```python
from build123d import *

# Parameters (mm, degrees)
SKETCH1_W                                = 60
SKETCH1_H                                = 50
BOSS_EXTRUDE1_DEPTH                      = 10
CUT_EXTRUDE1_DEPTH                       = 10
BOSS_EXTRUDE2_REACH                      = 80.74
CBORE_FOR_M3_PAN_HEAD_SCREW1_D           = 3.4
CBORE_FOR_M3_PAN_HEAD_SCREW1_CBORE_D     = 6.5
CBORE_FOR_M3_PAN_HEAD_SCREW1_CBORE_DEPTH = 3.3
M3X0_5_TAPPED_HOLE1_D                    = 2.6
M3X0_5_TAPPED_HOLE1_DEPTH                = 9
M3X0_5_TAPPED_HOLE1_TIP                  = 0.781118805
M3X0_5_TAPPED_HOLE2_D                    = 2.6
M3X0_5_TAPPED_HOLE2_DEPTH                = 9
M3X0_5_TAPPED_HOLE2_TIP                  = 0.781118805


with BuildPart() as part:
    # Sketch1 → Boss-Extrude1 (new body)
    with BuildSketch(Plane(origin=(0, 0, 0), x_dir=(1, 0, 0), z_dir=(0, 1, 0))):
        with Locations((30, 25)):
            Rectangle(SKETCH1_W, SKETCH1_H)
    extrude(amount=BOSS_EXTRUDE1_DEPTH)

    # Sketch2 → Cut-Extrude1 (cut)
    with BuildSketch(Plane(origin=(0, 10, 0), x_dir=(1, 0, 0), z_dir=(0, 1, 0))):
        with BuildLine():
            Line((38, 48), (38, 50))
            Line((38, 50), (44, 50))
            Line((44, 50), (44, 48))
            ThreePointArc((44, 48), (41, 45), (38, 48))
        make_face()
        with BuildLine():
            Line((10, 48), (10, 50))
            Line((10, 50), (16, 50))
            Line((16, 50), (16, 48))
            ThreePointArc((16, 48), (13, 45), (10, 48))
        make_face()
    extrude(amount=-CUT_EXTRUDE1_DEPTH, mode=Mode.SUBTRACT)

    # Sketch3 → Boss-Extrude2 (add, up to next)
    with BuildSketch(Plane(origin=(0, 0, 0), x_dir=(0, 0, -1), z_dir=(1, 0, 0)), mode=Mode.PRIVATE) as boss_extrude2_sk1:
        Polygon((45, 0), (50, 0), (50, 5), (45, 10), align=None)
    boss_extrude2_tool1 = extrude(boss_extrude2_sk1.sketch, amount=BOSS_EXTRUDE2_REACH, mode=Mode.PRIVATE) - part.part
    add(boss_extrude2_tool1.solids().sort_by_distance((0, 3.888889, -47.222222))[0])
    add(boss_extrude2_tool1.solids().sort_by_distance((0, 3.888889, -47.222222))[1])

    # CBORE for M3 Pan Head Screw1 (through all)
    with Locations(Plane(origin=(5, 10, -42), x_dir=(0, 0, 1), z_dir=(0, 1, 0))):
        with Locations((0, 0), (0, 44)):
            CounterBoreHole(CBORE_FOR_M3_PAN_HEAD_SCREW1_D / 2, CBORE_FOR_M3_PAN_HEAD_SCREW1_CBORE_D / 2, CBORE_FOR_M3_PAN_HEAD_SCREW1_CBORE_DEPTH)

    # M3x0.5 Tapped Hole1
    with Locations(Plane(origin=(60, 0, 0), x_dir=(0, 0, -1), z_dir=(1, 0, 0))):
        with Locations((34, 5), (9, 5)):
            Hole(M3X0_5_TAPPED_HOLE1_D / 2, depth=M3X0_5_TAPPED_HOLE1_DEPTH)
            with Locations((0, 0, -(M3X0_5_TAPPED_HOLE1_DEPTH + M3X0_5_TAPPED_HOLE1_TIP / 2))):  # 118° drill point
                Cone(0, M3X0_5_TAPPED_HOLE1_D / 2, M3X0_5_TAPPED_HOLE1_TIP, mode=Mode.SUBTRACT)

    # M3x0.5 Tapped Hole2
    with Locations(Plane.ZY):
        with Locations((-34, 5), (-9, 5)):
            Hole(M3X0_5_TAPPED_HOLE2_D / 2, depth=M3X0_5_TAPPED_HOLE2_DEPTH)
            with Locations((0, 0, -(M3X0_5_TAPPED_HOLE2_DEPTH + M3X0_5_TAPPED_HOLE2_TIP / 2))):  # 118° drill point
                Cone(0, M3X0_5_TAPPED_HOLE2_D / 2, M3X0_5_TAPPED_HOLE2_TIP, mode=Mode.SUBTRACT)


solid = part.part
```
Work out the finished part from the listing and answer in its coordinate system (mm). A direction names the side the tool comes from. Give positions to 0.01 mm unless a question says otherwise; leave off trailing zeros. Loops run counter-clockwise (first coordinate to the right, second up) from the corner with the lowest first, then second, coordinate; pieces in that order, holes last. Notation, with made-up numbers: M 63,88 L 95,88 A22 ccw 95,123 Z; hole C 64,-32 d6. An arc over 180 degrees is marked long. One line per item, written item: value. Start each with the question number.
1. Find the intervals of material crossed by probe 1 along X at (y, z) = (8.05, -42); probe 2 along Z at (x, y) = (57.25, 5); probe 3 along X at (y, z) = (2, -42), in increasing order.
2. Find section B-B (x = 53.5). Give the vertices of the cut face in (y, z).
3. Which of the six approach directions +Z, -Z, +X, -X, +Y, -Y give full straight-line access (tool end or side, diameter ignored) to faces 1 (the face through (30, 0, -25)), 2 (the face through (55.437, 3.847, -8.4)), 3 (the face through (47.6, 6.7, -40.6)), 4 (the face through (15.73, 9.19, -46.76)), 5 (the face through (4.6, 4.5, -10.2))?
4. Determine the mould class of faces 6 (the face through (30, 5, -50)), 7 (the face through (3.97, 3.3, -40.65)), 8 (the face through (60, 5, -25)), 9 (the face through (38.295, 9.188, -46.702)) for opening direction X: released by +X, released by -X, zero draft, split by the parting line, or undercut.
5. Find section A-A (z = -42). Give the vertices of the cut face in (x, y), and give its area (3 significant figures).
6. Each of these flat-tipped pins is pushed along its axis until it touches: P1, Ø4, axis at x = 5, z = -42, coming from the -Y side; P2, Ø5, axis at x = 5, z = -42.5, coming from the +Y side; P3, Ø2.5, axis at x = 5, z = -42, coming from the -Y side; P4, Ø2, axis at y = 5, z = -34, coming from the -X side. Where does it stop, or does it pass through?
7. Find section C-C (y = 8.5). Give the vertices of the cut face in (x, z), and give its area (3 significant figures).
Reported:
1. probe 1: x = 0 to 1.75, 8.25 to 45.75, 52.25 to 60
1. probe 2: z = -50 to -35.3, -32.7 to -10.3, -7.7 to 0
1. probe 3: x = 0 to 3.3, 6.7 to 47.3, 50.7 to 60
2. outline: M 0,-50 L 10,-50 L 10,0 L 0,0 Z; hole C 5,-34 d2.6; hole C 5,-9 d2.6
3. face 1: +Z, -Z, +X, -X, -Y
3. face 2: +X
3. face 3: +Y
3. face 4: -Z, +Y
3. face 5: -X
4. face 6: zero draft
4. face 7: undercut
4. face 8: released by +X
4. face 9: undercut
5. outline: M 0,0 L 3.3,0 L 3.3,6.7 L 1.75,6.7 L 1.75,10 L 0,10 Z; M 6.7,0 L 47.3,0 L 47.3,6.7 L 45.75,6.7 L 45.75,10 L 8.25,10 L 8.25,6.7 L 6.7,6.7 Z; M 50.7,0 L 60,0 L 60,10 L 52.25,10 L 52.25,6.7 L 50.7,6.7 Z
5. area: 512 mm²
6. P1: stops at y = 0
6. P2: stops at y = 6.7
6. P3: passes through
6. P4: stops at x = 9.18
7. outline: M 0,-50 L 10,-50 L 10,-48 A3 cw 10.4,-46.5 L 15.6,-46.5 A3 cw 16,-48 L 16,-50 L 38,-50 L 38,-48 A3 cw 38.4,-46.5 L 43.6,-46.5 A3 cw 44,-48 L 44,-50 L 60,-50 L 60,0 L 0,0 Z; hole C 5,-42 d6.5; hole C 49,-42 d6.5
7. area: 2,890 mm²
